Here's how the part is built. I have some questions about the finished solid (model axes, mm). A direction names the side the tool comes from. Round coordinates to 2 decimals unless told otherwise and drop trailing zeros. Answer as CSV lines item,"result".
from build123d import *

# Parameters (mm, degrees)
SKETCH_1_W           = 95
SKETCH_1_H           = 45
EXTRUDE_1_DEPTH      = 25
SHELL_1_T            = -4
FILLET_1_R           = 4.5
SKETCH_2_R           = 0.75
CUT_EXTRUDE_1_DEPTH  = 5
CUT_EXTRUDE_3_DEPTH  = 2.5
SKETCH_8_W           = 34
SKETCH_8_H           = 10
CUT_EXTRUDE_4_DEPTH  = 3
SKETCH_9_W           = 37
SKETCH_9_H           = 21
CUT_EXTRUDE_7_DEPTH  = 2
SKETCH_7_W           = 1
SKETCH_7_H           = 37
CUT_EXTRUDE_8_DEPTH  = 1
SKETCH_11_W          = 1
SKETCH_11_H          = 21
CUT_EXTRUDE_10_DEPTH = 1
SKETCH_12_W          = 1
SKETCH_12_H          = 21
CUT_EXTRUDE_11_DEPTH = 1
SKETCH_15_W          = 0.5
SKETCH_15_H          = 10
EXTRUDE_2_DEPTH      = 1
SKETCH_17_W          = 1.5
SKETCH_17_H          = 10
EXTRUDE_3_DEPTH      = 3
SKETCH_18_R          = 1.485
EXTRUDE_4_DEPTH      = 8
SKETCH_19_W          = 9.34
SKETCH_19_H          = 1.2
CUT_EXTRUDE_12_DEPTH = 10
FILLET_2_R           = 1
FILLET_3_R           = 1
FILLET_4_R           = 1
FILLET_5_R           = 1
SKETCH_20_W          = 2
SKETCH_20_H          = 6
EXTRUDE_5_DEPTH      = 5.8
EXTRUDE_6_DEPTH      = 17.3
EXTRUDE_7_DEPTH      = 14.3
SKETCH_26_W          = 15
SKETCH_26_H          = 4.9
EXTRUDE_8_DEPTH      = 2.4
SKETCH_27_W          = 12
SKETCH_27_H          = 4.4
SKETCH_27_H_2        = 4.5
EXTRUDE_9_DEPTH      = 4.6


with BuildPart() as part:
    # Эскиз1 → Бобышка-Вытянуть1 (new body)
    with BuildSketch(Plane(origin=(0, 0, 0), x_dir=(1, 0, 0), z_dir=(0, 1, 0))):
        with Locations((47.5, -22.5)):
            Rectangle(SKETCH_1_W, SKETCH_1_H)
    extrude(amount=EXTRUDE_1_DEPTH)

    # Оболочка1
    shell_1_openings = [part.faces().sort_by_distance(p)[0] for p in [
        (47.5, 25, 22.5),
    ]]
    offset(amount=SHELL_1_T, openings=shell_1_openings, kind=Kind.INTERSECTION)

    # Скругление1
    fillet_1_edges = [part.edges().sort_by_distance(p)[0] for p in [
        (47.5, 0, 0),
        (95, 0, 22.5),
        (47.5, 0, 45),
        (0, 0, 22.5),
        (0, 12.5, 0),
        (95, 12.5, 0),
        (95, 12.5, 45),
        (0, 12.5, 45),
    ]]
    fillet(fillet_1_edges, radius=FILLET_1_R)

    # Эскиз2 → Вырез-Вытянуть1 (cut)
    with BuildSketch(Plane(origin=(0, 25, 0), x_dir=(1, 0, 0), z_dir=(0, 1, 0))):
        with Locations((6, -2)):
            Circle(SKETCH_2_R)
        with BuildLine():
            ThreePointArc((2, -5.25), (2.530330086, -5.469669914), (2.75, -6))
            Line((2.75, -6), (2.75, -2.75))
            Line((2.75, -2.75), (6, -2.75))
            ThreePointArc((6, -2.75), (5.469669914, -2.530330086), (5.25, -2))
            Line((5.25, -2), (2, -2))
            Line((2, -2), (2, -5.25))
        make_face()
        with Locations((2, -6)):
            Circle(SKETCH_2_R)
        with Locations(Location((89, -43, 0), (0, 0, 270))):
            Circle(SKETCH_2_R)
        with Locations(Location((89, -2, 0), (0, 0, 270))):
            Circle(SKETCH_2_R)
        with Locations((2, -39)):
            Circle(SKETCH_2_R)
        with BuildLine():
            Line((2.75, -42.25), (2.75, -39))
            ThreePointArc((2.75, -39), (2.530330086, -39.530330086), (2, -39.75))
            Line((2, -39.75), (2, -43))
            Line((2, -43), (5.25, -43))
            ThreePointArc((5.25, -43), (5.469669914, -42.469669914), (6, -42.25))
            Line((6, -42.25), (2.75, -42.25))
        make_face()
        with Locations((6, -43)):
            Circle(SKETCH_2_R)
    extrude(amount=-CUT_EXTRUDE_1_DEPTH, mode=Mode.SUBTRACT)

    # Эскиз2<6> → Вырез-Вытянуть3 (cut)
    with BuildSketch(Plane(origin=(0, 25, 0), x_dir=(1, 0, 0), z_dir=(0, 1, 0))):
        with BuildLine():
            Line((2.75, -39), (2.75, -6))
            ThreePointArc((2.75, -6), (2.530330086, -6.530330086), (2, -6.75))
            Line((2, -6.75), (2, -38.25))
            ThreePointArc((2, -38.25), (2.530330086, -38.469669914), (2.75, -39))
        make_face()
        with BuildLine():
            ThreePointArc((6.75, -2), (6.530330086, -2.530330086), (6, -2.75))
            Line((6, -2.75), (89, -2.75))
            ThreePointArc((89, -2.75), (88.469669914, -2.530330086), (88.25, -2))
            Line((88.25, -2), (6.75, -2))
        make_face()
        with BuildLine():
            Line((89, -42.25), (6, -42.25))
            ThreePointArc((6, -42.25), (6.530330086, -42.469669914), (6.75, -43))
            Line((6.75, -43), (88.25, -43))
            ThreePointArc((88.25, -43), (88.469669914, -42.469669914), (89, -42.25))
        make_face()
    extrude(amount=-CUT_EXTRUDE_3_DEPTH, mode=Mode.SUBTRACT)

    # Эскиз8 → Вырез-Вытянуть4 (cut)
    with BuildSketch(Plane.ZY.offset(-91)):
        with Locations((22.5, 14.5)):
            Rectangle(SKETCH_8_W, SKETCH_8_H)
    extrude(amount=-CUT_EXTRUDE_4_DEPTH, mode=Mode.SUBTRACT)

    # Эскиз9 → Вырез-Вытянуть7 (cut)
    with BuildSketch(Plane.ZY.offset(-91)):
        with Locations((22.5, 14.5)):
            Rectangle(SKETCH_9_W, SKETCH_9_H)
    extrude(amount=-CUT_EXTRUDE_7_DEPTH, mode=Mode.SUBTRACT)

    # Эскиз7 → Вырез-Вытянуть8 (cut)
    with BuildSketch(Plane(origin=(0, 4, 0), x_dir=(1, 0, 0), z_dir=(0, 1, 0))):
        with Locations((90, -22.5)):
            Rectangle(SKETCH_7_W, SKETCH_7_H)
    extrude(amount=-CUT_EXTRUDE_8_DEPTH, mode=Mode.SUBTRACT)

    # Эскиз11 → Вырез-Вытянуть10 (cut)
    with BuildSketch(Plane.XY.offset(4)):
        with Locations((90, 14.5)):
            Rectangle(SKETCH_11_W, SKETCH_11_H)
    extrude(amount=-CUT_EXTRUDE_10_DEPTH, mode=Mode.SUBTRACT)

    # Эскиз12 → Вырез-Вытянуть11 (cut)
    with BuildSketch(Plane(origin=(0, 0, 41), x_dir=(-1, 0, 0), z_dir=(0, 0, -1))):
        with Locations((-90, 14.5)):
            Rectangle(SKETCH_12_W, SKETCH_12_H)
    extrude(amount=-CUT_EXTRUDE_11_DEPTH, mode=Mode.SUBTRACT)

    # Эскиз15 → Бобышка-Вытянуть2 (add)
    with BuildSketch(Plane.ZY.offset(-94)):
        with Locations((14.5, 14.5)):
            Rectangle(SKETCH_15_W, SKETCH_15_H)
        with Locations((22.5, 14.5)):
            Rectangle(SKETCH_15_W, SKETCH_15_H)
        with Locations((30.5, 14.5)):
            Rectangle(SKETCH_15_W, SKETCH_15_H)
    extrude(amount=EXTRUDE_2_DEPTH)

    # Эскиз17 → Бобышка-Вытянуть3 (add)
    with BuildSketch(Plane(origin=(0, 4, 0), x_dir=(1, 0, 0), z_dir=(0, 1, 0))):
        with Locations((61.75, -22.5)):
            Rectangle(SKETCH_17_W, SKETCH_17_H)
        Polygon((83, -3.75), (83, -4.75), (87, -4.75), (87, -8.75), (88.5, -8.75), (88.5, -3.75), align=None)
        Polygon((40.5, -3.75), (35.5, -3.75), (35.5, -8.75), (36.5, -8.75), (36.5, -4.75), (40.5, -4.75), align=None)
        Polygon((87, -36.25), (88.5, -36.25), (88.5, -41.25), (83, -41.25), (83, -40.25), (87, -40.25), align=None)
        Polygon((40.5, -40.25), (40.5, -41.25), (35.5, -41.25), (35.5, -36.25), (36.5, -36.25), (36.5, -40.25), align=None)
    extrude(amount=EXTRUDE_3_DEPTH)

    # Эскиз18 → Бобышка-Вытянуть4 (add)
    with BuildSketch(Plane(origin=(0, 4, 0), x_dir=(1, 0, 0), z_dir=(0, 1, 0))):
        with Locations(Location((33.4, -10.6, 0), (0, 0, 270))):
            Circle(SKETCH_18_R)
        with Locations(Location((33.4, -34.4, 0), (0, 0, 90))):
            Circle(SKETCH_18_R)
    extrude(amount=EXTRUDE_4_DEPTH)

    # Эскиз19 → Вырез-Вытянуть12 (cut)
    with BuildSketch(Plane.ZY):
        with Locations((22.5, 24.4)):
            Rectangle(SKETCH_19_W, SKETCH_19_H)
    extrude(amount=-CUT_EXTRUDE_12_DEPTH, mode=Mode.SUBTRACT)

    # Скругление2
    fillet_2_edges = [part.edges().sort_by_distance(p)[0] for p in [
        (1, 23.8, 27.17),
    ]]
    fillet(fillet_2_edges, radius=FILLET_2_R)

    # Скругление3
    fillet_3_edges = [part.edges().sort_by_distance(p)[0] for p in [
        (3.375, 23.8, 27.17),
    ]]
    fillet(fillet_3_edges, radius=FILLET_3_R)

    # Скругление4
    fillet_4_edges = [part.edges().sort_by_distance(p)[0] for p in [
        (3.375, 23.8, 17.83),
    ]]
    fillet(fillet_4_edges, radius=FILLET_4_R)

    # Скругление5
    fillet_5_edges = [part.edges().sort_by_distance(p)[0] for p in [
        (1, 23.8, 17.83),
    ]]
    fillet(fillet_5_edges, radius=FILLET_5_R)

    # Эскиз20 → Бобышка-Вытянуть5 (add)
    with BuildSketch(Plane(origin=(0, 4, 0), x_dir=(1, 0, 0), z_dir=(0, 1, 0))):
        Polygon((15.2, -10), (9.7, -10), (9.7, -15.5), (7.2, -15.5), (7.2, -7.5), (15.2, -7.5), align=None)
        Polygon((9.7, -29.5), (9.7, -35), (15.2, -35), (15.2, -37.5), (7.2, -37.5), (7.2, -29.5), align=None)
        with Locations((26.2, -16)):
            Rectangle(SKETCH_20_W, SKETCH_20_H)
        with Locations((26.2, -29)):
            Rectangle(SKETCH_20_W, SKETCH_20_H)
    extrude(amount=EXTRUDE_5_DEPTH)

    # Эскиз22 → Бобышка-Вытянуть6 (add)
    with BuildSketch(Plane(origin=(0, 4, 0), x_dir=(1, 0, 0), z_dir=(0, 1, 0))):
        Polygon((7.2, -7.5), (7.2, -11.5), (5.7, -11.5), (5.7, -6), (11.2, -6), (11.2, -7.5), align=None)
        Polygon((7.2, -33.5), (5.7, -33.5), (5.7, -39), (11.2, -39), (11.2, -37.5), (7.2, -37.5), align=None)
    extrude(amount=EXTRUDE_6_DEPTH)

    # Эскиз25 → Бобышка-Вытянуть7 (add)
    with BuildSketch(Plane(origin=(0, 7, 0), x_dir=(1, 0, 0), z_dir=(0, 1, 0))):
        Polygon((83, -4), (83, -4.75), (87, -4.75), (87, -8.75), (88.5, -8.75), (88.5, -4), align=None)
        Polygon((83, -40.25), (83, -41), (88.5, -41), (88.5, -36.25), (87, -36.25), (87, -40.25), align=None)
    extrude(amount=EXTRUDE_7_DEPTH)

    # Эскиз26 → Бобышка-Вытянуть8 (add)
    with BuildSketch(Plane.XZ):
        with Locations((41.5, 22.5)):
            Rectangle(SKETCH_26_W, SKETCH_26_H)
    extrude(amount=EXTRUDE_8_DEPTH)

    # Эскиз27 → Бобышка-Вытянуть9 (add)
    with BuildSketch(Plane.XZ):
        with Locations((55, 28.6)):
            Rectangle(SKETCH_27_W, SKETCH_27_H)
        with Locations((55, 16.45)):
            Rectangle(SKETCH_27_W, SKETCH_27_H_2)
    extrude(amount=EXTRUDE_9_DEPTH)


solid = part.part
Item 1: Suppose I cut it at A-A, the plane y = 14.75. State how many separate pieces and enclosed holes the cut face has, then the cut area to 3 significant figures.
Results found:
separate pieces,"3"
enclosed holes,"1"
area,"979 mm²"
Item 2: I need wall thicknesses on L1, parallel to Z at x = 89, y = 22.75; L2, parallel to X at y = 23.4, z = 6. Which ranges of each line are inside material? Lowest first, please.
Results found:
L1,"z = 0 to 1.25, 2.75 to 4, 41 to 42.25, 43.75 to 45"
L2,"x = 0 to 1.25, 2.75 to 4, 93 to 95"
Item 3: Will these pins go through, and if not, where does the flat tip stop? pin 1 (4 mm diameter, centred on x = 33.5, z = 25.5, fed in from -Y); pin 2 (0.6 mm diameter, centred on x = 0.5, z = 21, fed in from +Y); pin 3 (0.5 mm diameter, centred on y = 3.5, z = 20.5, fed in from +X).
Results found:
pin 1,"stops at y = -2.4"
pin 2,"stops at y = 23.8"
pin 3,"stops at x = 94.94"
Item 4: For faces 4 (the flat face through (61, -2, 29)), 5 (the flat face through (94, 15, 18)), 6 (the flat face through (88.5, 13, 39)), which set-ups out of +Z, -Z, +X, -X, +Y, -Y let a thin tool reach every point of the face, with its end or its side?
Results found:
face 4,"+Z, -Z, +X, -Y"
face 5,"none"
face 6,"+Y"
Item 5: If we mould it in two halves opening along Z, with no side actions, what happens to faces 1 (the flat face through (46, 4, 22)), 2 (the flat face through (47, 15, 0)), 3 (the flat face through (55, -4.6, 29))? For each: pulls with the +Z half, pulls with the -Z half, needs draft (parallel to the pull), parting line crosses it, or undercut.
Results found:
face 1,"undercut"
face 2,"pulls with the -Z half"
face 3,"needs draft"
